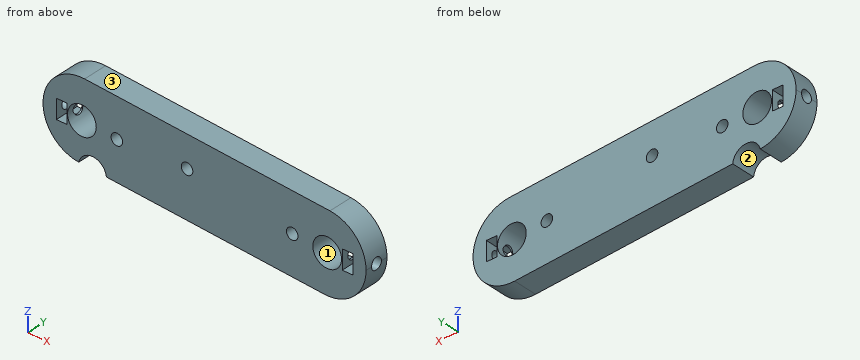
from build123d import *

# Parameters (mm, degrees)
ESBO_O2_R                  = 4.1
ESBO_O2_R_2                = 1.65
ESBO_O2_W                  = 3
ESBO_O2_H                  = 5.5
RESSALTO_EXTRUS_O1_DEPTH   = 7
ESBO_O3_W                  = 117.766713874
ESBO_O3_H                  = 105.694955048
CORTE_EXTRUS_O1_DEPTH      = 1
CORTE_EXTRUS_O1_DEPTH_BACK = 8
ESBO_O4_R                  = 1.65
CORTE_EXTRUS_O2_DEPTH      = 7.8
CORTE_EXTRUS_O2_DEPTH_BACK = 2
ESBO_O5_R                  = 1.65
CORTE_EXTRUS_O3_DEPTH      = 10
CORTE_EXTRUS_O3_DEPTH_BACK = 2
ESBO_O6_R                  = 4
CORTE_EXTRUS_O4_DEPTH      = 1.0000001
CORTE_EXTRUS_O4_DEPTH_BACK = 8.0000001


with BuildPart() as part:
    # Esboço2 → Ressalto-extrusão1 (new body)
    with BuildSketch(Plane(origin=(0, 0, 0), x_dir=(1, 0, 0), z_dir=(0, 1, 0))):
        with BuildLine():
            Line((-0.790842255, 46.071791568), (69.209157745, 51.071791568))
            ThreePointArc((69.209157745, 51.071791568), (77.564114323, 48.123679863), (81.1, 40))
            Line((81.1, 40), (81.1, -40))
            ThreePointArc((81.1, -40), (77.564114323, -48.123679863), (69.209157745, -51.071791568))
            Line((69.209157745, -51.071791568), (-0.790842255, -46.071791568))
            ThreePointArc((-0.790842255, -46.071791568), (-8.123679863, -42.564114323), (-11.1, -35))
            Line((-11.1, -35), (-11.1, 35))
            ThreePointArc((-11.1, 35), (-8.123679863, 42.564114323), (-0.790842255, 46.071791568))
        make_face()
        with Locations((0, 35)):
            Circle(ESBO_O2_R, mode=Mode.SUBTRACT)
        with Locations((70, 40)):
            Circle(ESBO_O2_R, mode=Mode.SUBTRACT)
        with Locations((70, -40)):
            Circle(ESBO_O2_R, mode=Mode.SUBTRACT)
        with Locations((0, -35)):
            Circle(ESBO_O2_R, mode=Mode.SUBTRACT)
        with Locations((9.974586998, 35.7124705)):
            Circle(ESBO_O2_R_2, mode=Mode.SUBTRACT)
        with Locations((60.025413002, 39.2875295)):
            Circle(ESBO_O2_R_2, mode=Mode.SUBTRACT)
        with Locations((9.974586998, -35.7124705)):
            Circle(ESBO_O2_R_2, mode=Mode.SUBTRACT)
        with Locations((60.025413002, -39.2875295)):
            Circle(ESBO_O2_R_2, mode=Mode.SUBTRACT)
        with Locations((30, 35)):
            Circle(ESBO_O2_R_2, mode=Mode.SUBTRACT)
        with Locations((30, -35)):
            Circle(ESBO_O2_R_2, mode=Mode.SUBTRACT)
        with Locations((-5.8, 35)):
            Rectangle(ESBO_O2_W, ESBO_O2_H, mode=Mode.SUBTRACT)
        with Locations((75.8, 40)):
            Rectangle(ESBO_O2_W, ESBO_O2_H, mode=Mode.SUBTRACT)
        with Locations((75.8, -40)):
            Rectangle(ESBO_O2_W, ESBO_O2_H, mode=Mode.SUBTRACT)
        with Locations((-5.8, -35)):
            Rectangle(ESBO_O2_W, ESBO_O2_H, mode=Mode.SUBTRACT)
    extrude(amount=RESSALTO_EXTRUS_O1_DEPTH)

    # Esboço3 → Corte-extrusão1 (cut, two sides)
    with BuildSketch(Plane(origin=(0, 7, 0), x_dir=(1, 0, 0), z_dir=(0, 1, 0))) as corte_extrus_o1_sk:
        with Locations((40.401748759, 0)):
            Rectangle(ESBO_O3_W, ESBO_O3_H)
        with BuildLine():
            Line((0.790842255, 23.928208432), (70.790842255, 28.928208432))
            ThreePointArc((70.790842255, 28.928208432), (81.071791568, 40.790842255), (69.209157745, 51.071791568))
            Line((69.209157745, 51.071791568), (-0.790842255, 46.071791568))
            ThreePointArc((-0.790842255, 46.071791568), (-11.071791568, 34.209157745), (0.790842255, 23.928208432))
        make_face(mode=Mode.SUBTRACT)
    extrude(amount=CORTE_EXTRUS_O1_DEPTH, mode=Mode.SUBTRACT)
    extrude(corte_extrus_o1_sk.sketch, amount=-CORTE_EXTRUS_O1_DEPTH_BACK, mode=Mode.SUBTRACT)

    # Esboço4 → Corte-extrusão2 (cut, two sides)
    with BuildSketch(Plane.ZY.offset(4.3)) as corte_extrus_o2_sk:
        with Locations((-35, 3.5)):
            Circle(ESBO_O4_R)
    extrude(amount=CORTE_EXTRUS_O2_DEPTH, mode=Mode.SUBTRACT)
    extrude(corte_extrus_o2_sk.sketch, amount=-CORTE_EXTRUS_O2_DEPTH_BACK, mode=Mode.SUBTRACT)

    # Esboço5 → Corte-extrusão3 (cut, two sides)
    with BuildSketch(Plane(origin=(74.3, 0, 0), x_dir=(0, 0, -1), z_dir=(1, 0, 0))) as corte_extrus_o3_sk:
        with Locations((40, 3.5)):
            Circle(ESBO_O5_R)
    extrude(amount=CORTE_EXTRUS_O3_DEPTH, mode=Mode.SUBTRACT)
    extrude(corte_extrus_o3_sk.sketch, amount=-CORTE_EXTRUS_O3_DEPTH_BACK, mode=Mode.SUBTRACT)

    # Esboço6 → Corte-extrusão4 (cut, two sides)
    with BuildSketch(Plane(origin=(0, 7, 0), x_dir=(1, 0, 0), z_dir=(0, 1, 0))) as corte_extrus_o4_sk:
        with Locations((3, 47)):
            Circle(ESBO_O6_R)
    extrude(amount=CORTE_EXTRUS_O4_DEPTH, mode=Mode.SUBTRACT)
    extrude(corte_extrus_o4_sk.sketch, amount=-CORTE_EXTRUS_O4_DEPTH_BACK, mode=Mode.SUBTRACT)


solid = part.part
Here's how the part is built. I have some questions about the finished solid (model axes, mm). Face numbers are marked on the shaded views. Coordinates: 2 decimals unless noted, no trailing zeros. Loops run counter-clockwise (first coordinate to the right, second up) from the corner with the lowest first, then second, coordinate; pieces in that order, holes last. Notation, with made-up numbers: (-2.5, 18) -> (53.5, 18) arc R19 ccw to (53.5, 50) -> close; hole circle Ø5 at (14.25, 38.5). An arc over 180 degrees is marked (long way). Use one line per item in the form item = value. Start each with the question number.
(1) If we section it at C-C (x = 70): Please give me the cut outline in (y, z), then the cut area to 3 significant figures.
(2) Please list where these lines run through material, in increasing order: line 1 along X through (y, z) = (3, -43.5); line 2 along Y through (x, z) = (80, -40); line 3 along X through (y, z) = (3.75, -35).
(3) We'd pull the mould along Z, two halves only. Please class the marked faces 1, 2 and 3: pulls with the +Z half, pulls with the -Z half, needs draft (parallel to the pull), parting line crosses it, or undercut.
(4) Will these pins go through, and if not, where does the flat tip stop? pin 1 (1 mm diameter, centred on y = 6, z = -31.5, fed in from -X); pin 2 (1.5 mm diameter, centred on x = 67.5, y = 4.5, fed in from +Z); pin 3 (9.5 mm diameter, centred on x = 70, z = -40, fed in from -Y); pin 4 (2.5 mm diameter, centred on x = 75.5, y = 3.5, fed in from +Z).
(5) If we section it at A-A (x = 0): Please give me the cut outline in (y, z), then the cut area to 3 significant figures.
(6) If we section it at D-D (z = -26): Please give me the cut outline in (x, y), then the cut area to 3 significant figures.
Verdict:
q1.outline = (0, -51.1) -> (7, -51.1) -> (7, -44.1) -> (0, -44.1) -> close; (0, -35.9) -> (7, -35.9) -> (7, -28.87) -> (0, -28.87) -> close
q1.area = 98.2 mm²
q2.line_1 = -7.14 to 1.06, 4.94 to 67.86, 72.14 to 80.53
q2.line_2 = 0 to 1.85, 5.15 to 7
q2.line_3 = 4.1 to 8.49, 11.46 to 28.35, 31.65 to 79.91
q3.face_1 = undercut
q3.face_2 = pulls with the -Z half
q3.face_3 = pulls with the +Z half
q4.pin_1 = -10.69
q4.pin_2 = -28.64
q4.pin_3 = 0
q4.pin_4 = -29.75
q5.outline = (0, -44.35) -> (7, -44.35) -> (7, -39.1) -> (0, -39.1) -> close; (0, -30.9) -> (7, -30.9) -> (7, -23.9) -> (0, -23.9) -> close
q5.area = 85.8 mm²
q6.outline = (-6.5, 0) -> (29.8, 0) -> (29.8, 7) -> (-6.5, 7) -> close
q6.area = 254 mm²
